Design review of the part built by this model. Coordinates are the model's own, in mm. Round coordinates to 2 decimals unless told otherwise and drop trailing zeros. Write each loop counter-clockwise with the first axis right and the second up, starting at its lowest first coordinate (ties: lowest second). Pieces come first, ordered by that corner, then holes. Notation, with made-up numbers: M -0.75,-4.5 L 17.25,-4.5 A21 cw 17.25,18.5 Z; hole C -29.75,38 d3. An arc over 180 degrees is marked long. Use CSV: the item, a comma, the result in double quotes.
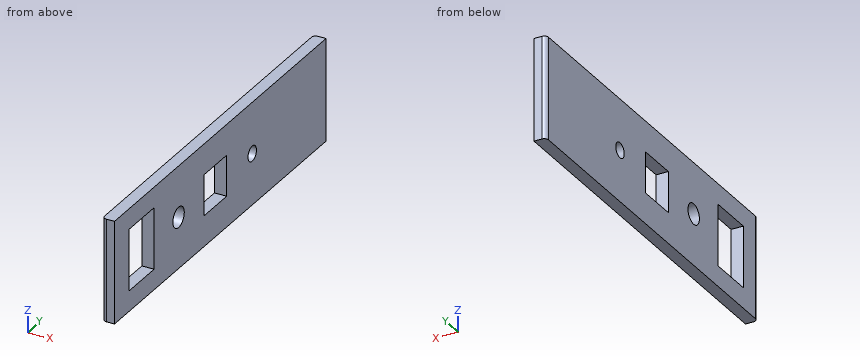
from build123d import *

# Parameters (mm, degrees)
F0_W     = 185.6
F0_H     = 50
F1_DEPTH = 6
F2_W     = 22.1
F2_H     = 30
F3_DEPTH = 6
F4_R     = 5
F5_DEPTH = 6
F6_W     = 20
F6_H     = 20
F7_DEPTH = 6
F8_R     = 3.7
F9_DEPTH = 6
F10_R    = 2


with BuildPart() as f1:
    # F0 (on Right) → F1 (new body)
    with BuildSketch(Plane.YZ):
        Rectangle(F0_W, F0_H)
    extrude(amount=F1_DEPTH)

    # F2 (on face) → F3 (cut, through all)
    with BuildSketch(Plane.YZ.offset(6)):
        with Locations((-69.095318, 0)):
            Rectangle(F2_W, F2_H)
    extrude(amount=-F3_DEPTH, mode=Mode.SUBTRACT)

    # F4 (on face) → F5 (cut, through all)
    with BuildSketch(Plane.YZ.offset(6)):
        with Locations((-36.594901, 0)):
            Circle(F4_R)
    extrude(amount=-F5_DEPTH, mode=Mode.SUBTRACT)

    # F6 (on face) → F7 (cut, through all)
    with BuildSketch(Plane.YZ.offset(6)):
        with Locations((-4.348571, 0)):
            Rectangle(F6_W, F6_H)
    extrude(amount=-F7_DEPTH, mode=Mode.SUBTRACT)

    # F8 (on face) → F9 (cut, through all)
    with BuildSketch(Plane.YZ.offset(6)):
        with Locations((28.03257, 0)):
            Circle(F8_R)
    extrude(amount=-F9_DEPTH, mode=Mode.SUBTRACT)

    # F10
    f10_edges = [f1.edges().sort_by_distance(p)[0] for p in [
        (0, 92.8, 0),
        (0, -92.8, 0),
    ]]
    fillet(f10_edges, radius=F10_R)


solid = f1.part
1) Wall thickness on line 1 along Y through (x, z) = (3.6, -8); line 2 along Z through (x, y) = (2.9, -61); line 3 along Z through (x, y) = (2.8, 4): over which ranges is each line inside the solid? List them lowest first. Write a range as [from, to].
Answers:
line 1,"[-92.8, -80.15], [-58.05, -14.35], [5.65, 92.8]"
line 2,"[-25, -15], [15, 25]"
line 3,"[-25, -10], [10, 25]"
2) For pin 1 Ø8 at (y, z) = (-36.59, 0) entering from -X, flat-tipped, find the tip position at first contact; note if it passes through.
Answers:
pin 1,"through"
3) Add section B-B on z = 0. Write out the cut boundary in (x, y).
Answers:
outline,"M 0,-90.8 A2 ccw 2,-92.8 L 6,-92.8 L 6,-80.15 L 0,-80.15 Z; M 0,-58.05 L 6,-58.05 L 6,-41.59 L 0,-41.59 Z; M 0,-31.59 L 6,-31.59 L 6,-14.35 L 0,-14.35 Z; M 0,5.65 L 6,5.65 L 6,24.33 L 0,24.33 Z; M 0,31.73 L 6,31.73 L 6,92.8 L 2,92.8 A2 ccw 0,90.8 Z"
4) Add section A-A on y = -7. Write out the cut boundary in (x, z).
Answers:
outline,"M 0,-25 L 6,-25 L 6,-10 L 0,-10 Z; M 0,10 L 6,10 L 6,25 L 0,25 Z"
5) Add section C-C on y = -72.5. Write out the cut boundary in (x, z), then the cut area to 3 significant figures.
Answers:
outline,"M 0,-25 L 6,-25 L 6,-15 L 0,-15 Z; M 0,15 L 6,15 L 6,25 L 0,25 Z"
area,"120 mm²"
